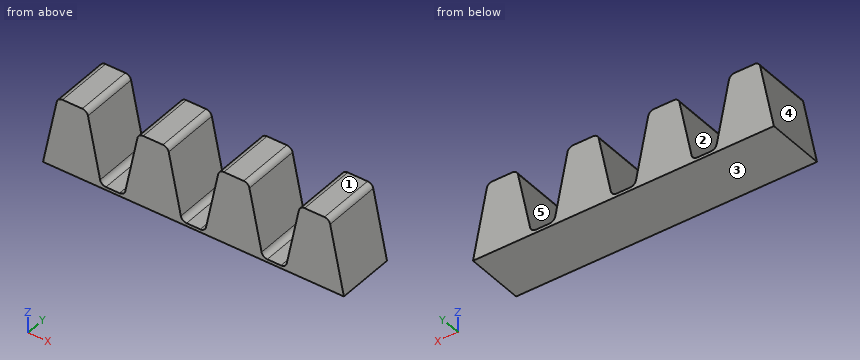
```python
from build123d import *

# Parameters (mm, degrees)
F1_DEPTH = 50.8
F2_R     = 5.08
F3_R     = 5.08
F4_R     = 5.08
F5_R     = 5.08
F6_R     = 5.08
F7_R     = 5.08
F8_R     = 5.08
F9_R     = 5.08
F10_R    = 5.08
F11_R    = 5.08
F12_R    = 5.08
F13_R    = 5.08
F14_R    = 5.08
F15_R    = 5.08


with BuildPart() as f1:
    # F0 (on Front) → F1 (new body)
    with BuildSketch(Plane.XZ):
        Polygon((-107.95, 34.678186), (-120.65, -27.538854), (-69.85, -27.538854), (-70.377374, -24.955261), (-82.55, 34.678186), align=None)
        Polygon((-70.377374, -24.955261), (-69.85, -27.538854), (-50.8, -27.538854), (-50.272626, -24.955261), align=None)
        Polygon((-50.272626, -24.955261), (-50.8, -27.538854), (0, -27.538854), (-0.527374, -24.955261), (-12.7, 34.678186), (-38.1, 34.678186), align=None)
        Polygon((-0.527374, -24.955261), (0, -27.538854), (19.05, -27.538854), (19.577374, -24.955261), align=None)
        Polygon((19.577374, -24.955261), (19.05, -27.538854), (69.85, -27.538854), (69.322626, -24.955261), (57.15, 34.678186), (31.75, 34.678186), align=None)
        Polygon((69.322626, -24.955261), (69.85, -27.538854), (88.9, -27.538854), (89.427374, -24.955261), align=None)
        Polygon((89.427374, -24.955261), (88.9, -27.538854), (139.7, -27.538854), (127, 34.678186), (101.6, 34.678186), align=None)
    extrude(amount=F1_DEPTH)

    # F2
    f2_edges = [f1.edges().sort_by_distance(p)[0] for p in [
        (-50.272626, -25.4, -24.955261),
    ]]
    fillet(f2_edges, radius=F2_R)

    # F3
    f3_edges = [f1.edges().sort_by_distance(p)[0] for p in [
        (-70.377374, -25.4, -24.955261),
    ]]
    fillet(f3_edges, radius=F3_R)

    # F4
    f4_edges = [f1.edges().sort_by_distance(p)[0] for p in [
        (19.577374, -25.4, -24.955261),
    ]]
    fillet(f4_edges, radius=F4_R)

    # F5
    f5_edges = [f1.edges().sort_by_distance(p)[0] for p in [
        (-0.527374, -25.4, -24.955261),
    ]]
    fillet(f5_edges, radius=F5_R)

    # F6
    f6_edges = [f1.edges().sort_by_distance(p)[0] for p in [
        (69.322626, -25.4, -24.955261),
    ]]
    fillet(f6_edges, radius=F6_R)

    # F7
    f7_edges = [f1.edges().sort_by_distance(p)[0] for p in [
        (89.427374, -25.4, -24.955261),
    ]]
    fillet(f7_edges, radius=F7_R)

    # F8
    f8_edges = [f1.edges().sort_by_distance(p)[0] for p in [
        (-82.55, -25.4, 34.678186),
    ]]
    fillet(f8_edges, radius=F8_R)

    # F9
    f9_edges = [f1.edges().sort_by_distance(p)[0] for p in [
        (-38.1, -25.4, 34.678186),
    ]]
    fillet(f9_edges, radius=F9_R)

    # F10
    f10_edges = [f1.edges().sort_by_distance(p)[0] for p in [
        (-12.7, -25.4, 34.678186),
    ]]
    fillet(f10_edges, radius=F10_R)

    # F11
    f11_edges = [f1.edges().sort_by_distance(p)[0] for p in [
        (31.75, -25.4, 34.678186),
    ]]
    fillet(f11_edges, radius=F11_R)

    # F12
    f12_edges = [f1.edges().sort_by_distance(p)[0] for p in [
        (57.15, -25.4, 34.678186),
    ]]
    fillet(f12_edges, radius=F12_R)

    # F13
    f13_edges = [f1.edges().sort_by_distance(p)[0] for p in [
        (101.6, -25.4, 34.678186),
    ]]
    fillet(f13_edges, radius=F13_R)

    # F14
    f14_edges = [f1.edges().sort_by_distance(p)[0] for p in [
        (127, -25.4, 34.678186),
    ]]
    fillet(f14_edges, radius=F14_R)

    # F15
    f15_edges = [f1.edges().sort_by_distance(p)[0] for p in [
        (-107.95, -25.4, 34.678186),
    ]]
    fillet(f15_edges, radius=F15_R)


solid = f1.part
```
For this review, take the finished solid that the model builds, in its own axes (mm). Face numbers are marked on the shaded views. A direction names the side the tool comes from. Give positions to 0.01 mm unless a question says otherwise; leave off trailing zeros. Write each loop counter-clockwise with the first axis right and the second up, starting at its lowest first coordinate (ties: lowest second). Pieces come first, ordered by that corner, then holes. Notation, with made-up numbers: M 4,-10.5 L 22,-10.5 A16 ccw 22,11.5 Z; hole C 47,49.25 d6. An arc over 180 degrees is marked long. Answer as a JSON object with one key per item and string values. Group by question number.
Item 1: Consider section D-D on x = -63.5. Write out the cut boundary in (y, z), plus the area to 3 significant figures.
Item 2: Tool access review of the marked faces 1 and 2: name each direction out of +Z, -Z, +X, -X, +Y, -Y from which nothing blocks a thin tool from reaching the whole face with its end or side.
Item 3: Consider section A-A on z = 11. Write out the cut boundary in (x, y), plus the area to 3 significant figures.
Item 4: Draft analysis for pull direction X (two halves, no side actions). For the marked faces 3, 4 and 5, state which applies: +X half, -X half, draft (parallel to the pull), parting line (faces both ways), or undercut.
Item 5: For pin 1 Ø9.5 at (x, y) = (79.5, -18) entering from +Z; pin 2 Ø10 at (y, z) = (-17, 19) entering from +X; pin 3 Ø1.5 at (y, z) = (-23.5, 10) entering from -X, all flat-tipped, find the tip position at first contact; note any pin that passes through.
Item 6: For probe 1 along X at (y, z) = (-7.5, 18); probe 2 along X at (y, z) = (-8.5, 21.5); probe 3 along Z at (x, y) = (79, -45), list the stretches that pass through material, from the lowest coordinate up. Write a range as [from, to].
Item 7: Consider section C-C on z = -18. Write out the cut boundary in (x, y).
Check result:
{
 "1": {"outline": "M -50.8,-27.54 L 0,-27.54 L 0,-24.96 L -50.8,-24.96 Z", "area": "131 mm^2"},
 "2": {"face 1": "+Z, +X, -X, +Y, -Y", "face 2": "+Z, +Y, -Y"},
 "3": {"outline": "M -112.78,-50.8 L -77.72,-50.8 L -77.72,0 L -112.78,0 Z; M -42.93,-50.8 L -7.87,-50.8 L -7.87,0 L -42.93,0 Z; M 26.92,-50.8 L 61.98,-50.8 L 61.98,0 L 26.92,0 Z; M 96.77,-50.8 L 131.83,-50.8 L 131.83,0 L 96.77,0 Z", "area": "7,130 mm^2"},
 "4": {"face 3": "draft", "face 4": "-X half", "face 5": "undercut"},
 "5": {"pin 1": "stops at z = -24.96", "pin 2": "stops at x = 131.22", "pin 3": "stops at x = -113.14"},
 "6": {"probe 1": "x = [-111.35, -79.15], [-41.5, -9.3], [28.35, 60.55], [98.2, 130.4]", "probe 2": "x = [-110.64, -79.86], [-40.79, -10.01], [29.06, 59.84], [98.91, 129.69]", "probe 3": "z = [-27.54, -24.96]"},
 "7": {"outline": "M -118.7,-50.8 L -71.8,-50.8 L -71.8,0 L -118.7,0 Z; M -48.85,-50.8 L -1.95,-50.8 L -1.95,0 L -48.85,0 Z; M 21,-50.8 L 67.9,-50.8 L 67.9,0 L 21,0 Z; M 90.85,-50.8 L 137.75,-50.8 L 137.75,0 L 90.85,0 Z"}
}
